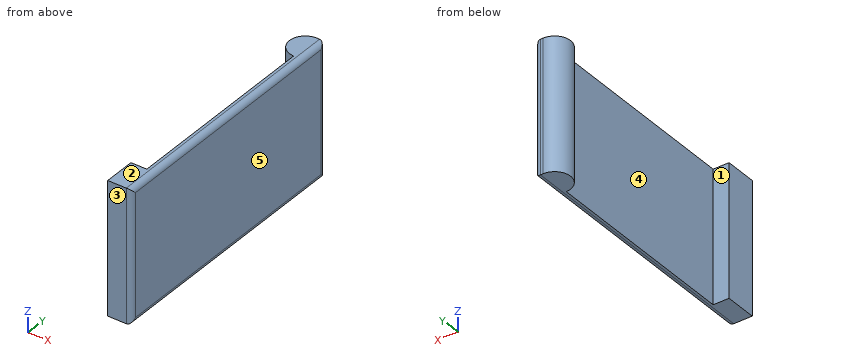
```python
from build123d import *

# Parameters (mm, degrees)
PAD_DEPTH = 25
FILLET_R  = 1


with BuildPart() as part:
    # Sketch → Pad (new body)
    with BuildSketch(Plane.XY):
        with BuildLine():
            Line((1.5, -44), (1.5, 6))
            Line((1.5, 6), (0, 6))
            ThreePointArc((0, 6), (-3, 3), (0, 0))
            Line((0, 0), (0, -38))
            Line((0, -38), (-3, -38))
            Line((-3, -38), (-3, -44))
            Line((1.5, -44), (-3, -44))
        make_face()
    extrude(amount=PAD_DEPTH)

    # Fillet
    fillet_edges = [part.edges().sort_by_distance(p)[0] for p in [
        (1.5, -44, 12.5),
        (1.5, 6, 12.5),
        (1.5, -19, 0),
        (1.5, -19, 25),
    ]]
    fillet(fillet_edges, radius=FILLET_R)


solid = part.part
```
Build history of the part. All positions in model axes, mm. Face numbers are marked on the shaded views. A direction names the side the tool comes from. Give positions to 0.01 mm unless a question says otherwise; leave off trailing zeros. Loops run counter-clockwise (first coordinate to the right, second up) from the corner with the lowest first, then second, coordinate; pieces in that order, holes last. Notation, with made-up numbers: (-10, 46) -> (37, 46) arc R19 ccw to (37, 79) -> close; hole circle Ø5 at (86, -30.5). An arc over 180 degrees is marked (long way). One line per question, with ' | ' between items. Start each with the question number.
1) Cut at B-B (z = 11). Give the cut face in (x, y).
2) Cut at A-A (x = -2.5). Give the cut face in (y, z).
3) Cut at C-C (y = -23). Give the cut face in (x, z).
4) Pin check, flat tips, straight feed: pin 1 (2 mm diameter, centred on x = 0.5, y = -32.5, fed in from -Z); pin 2 (1.5 mm diameter, centred on y = -1.5, z = 15.5, fed in from -X). Stop position of each tip, or through.
5) Probe L1, parallel to Y at x = -0.15, z = 16; L2, parallel to X at y = -15, z = 2.5; L3, parallel to Z at x = 0.6, y = -8. List the from-to ranges inside material, lowest first.
6) 3-axis set-ups, long thin cutter, end or side, ignore diameter. For the marked faces 4 and 5: which of +Z, -Z, +X, -X, +Y, -Y reach the whole face in a straight line?
7) Two-plate mould, pull along Y, no slides. Class the marked faces 1, 2 and 3: released by +Y, released by -Y, zero draft, split by the parting line, or undercut.
Return value:
1) outline: (-3, -44) -> (0.5, -44) arc R1 ccw to (1.5, -43) -> (1.5, 5) arc R1 ccw to (0.5, 6) -> (0, 6) arc R3 ccw to (0, 0) -> (0, -38) -> (-3, -38) -> close
2) outline: (-44, 0) -> (-38, 0) -> (-38, 25) -> (-44, 25) -> close; (1.34, 0) -> (4.66, 0) -> (4.66, 25) -> (1.34, 25) -> close
3) outline: (0, 0) -> (0.5, 0) arc R1 ccw to (1.5, 1) -> (1.5, 24) arc R1 ccw to (0.5, 25) -> (0, 25) -> close
4) pin 1: z = 0 | pin 2: x = 0
5) L1: -44 to -38, 0 to 6 | L2: 0 to 1.5 | L3: 0.01 to 24.99
6) face 4: +Z, -Z, -X | face 5: +Z, -Z, +X, +Y, -Y
7) face 1: undercut | face 2: zero draft | face 3: released by -Y
